The listing builds one solid part. Answer for the finished solid, in the listing's coordinates (mm). A direction names the side the tool comes from. Round coordinates to 2 decimals unless told otherwise and drop trailing zeros. Order: outer loops, then holes, each group sorted by start corner. A loop starts at its lowest first (then second) coordinate and runs counter-clockwise, first axis right, second up. Notation, with made-up numbers: (-34.5, -2.5) -> (-22.5, -2.5) arc R13 ccw to (-22.5, 17.5) -> close; hole circle Ø3 at (75.5, 30.25). An arc over 180 degrees is marked (long way). Answer in a Markdown table with one row per item. Add a question column.
```python
from build123d import *

# Parameters (mm, degrees)
SKETCH1_W           = 36
SKETCH1_H           = 29
BOSS_EXTRUDE1_DEPTH = 1.5
FILLET1_R           = 0.8
SKETCH2_W           = 20
SKETCH2_H           = 1
BOSS_EXTRUDE2_DEPTH = 3


with BuildPart() as part:
    # Sketch1 → Boss-Extrude1 (new body)
    with BuildSketch(Plane(origin=(0, 0, 0), x_dir=(1, 0, 0), z_dir=(0, 1, 0))):
        with Locations((18, -14.5)):
            Rectangle(SKETCH1_W, SKETCH1_H)
    extrude(amount=BOSS_EXTRUDE1_DEPTH)

    # Fillet1
    fillet1_edges = [part.edges().sort_by_distance(p)[0] for p in [
        (0, 0.75, 0),
        (36, 0.75, 0),
        (36, 0.75, 29),
        (0, 0.75, 29),
    ]]
    fillet(fillet1_edges, radius=FILLET1_R)

    # Sketch2 → Boss-Extrude2 (add)
    with BuildSketch(Plane(origin=(0, 1.5, 0), x_dir=(1, 0, 0), z_dir=(0, 1, 0))):
        with Locations((18, -2)):
            Rectangle(SKETCH2_W, SKETCH2_H)
        with Locations((18, -27)):
            Rectangle(SKETCH2_W, SKETCH2_H)
    extrude(amount=BOSS_EXTRUDE2_DEPTH)


solid = part.part
```
Item 1: Find the intervals of material crossed by probe 1 along Z at (x, y) = (26, 2.6); probe 2 along X at (y, z) = (2.3, 27.25); probe 3 along Y at (x, z) = (18, 4), in increasing order. Write a range as [from, to].
Item 2: The part is cut by section A-A, the plane y = 2.75. Give the vertices of the cut face in (x, z).
Item 3: A tool of negligible diameter and unlimited length cuts with its end or side. For faces 1 (the face through (28, 3, 27)), 2 (the face through (18, 0, 14)), 3 (the face through (35.77, 0.76, 0.24)), 4 (the face through (18, 3, 2.5)), 5 (the face through (8, 3, 2)), from which of +Z, -Z, +X, -X, +Y, -Y can it reach the whole face along a straight path? Write none if from no direction.
Item 4: For a pull along Z with two mould halves and no side action, classify faces 6 (the face through (18, 1.5, 14)), 7 (the face through (18, 3, 27.5)), 8 (the face through (0, 1, 15)) as released by +Z, released by -Z, zero draft, split by the parting line, or undercut.
Item 5: The part is cut by section C-C, the plane z = 7. Give the vertices of the cut face in (x, y), and give its area (3 significant figures).
Item 6: The part is cut by section D-D, the plane x = 30. Give the vertices of the cut face in (y, z).
Item 7: Flat-ended cylindrical pins translate along their axes: P1, Ø0.8, axis at y = 3.5, z = 27, coming from the +X side; P2, Ø2.5, axis at x = 20, y = 2.5, coming from the -Z side; P3, Ø6, axis at x = 15, z = 13, coming from the +Y side; P4, Ø0.9, axis at x = 15.5, y = 2.5, coming from the +Z side. Find the tip coordinate at first contact, or state that the pin passes through.
Item 8: The part is cut by section B-B, the plane x = 14. Give the vertices of the cut face in (y, z).
Resolved:
| question | item | result |
|---|---|---|
| 1 | probe 1 | [1.5, 2.5], [26.5, 27.5] |
| 1 | probe 2 | [8, 28] |
| 1 | probe 3 | [0, 1.5] |
| 2 | outline | (8, 1.5) -> (28, 1.5) -> (28, 2.5) -> (8, 2.5) -> close; (8, 26.5) -> (28, 26.5) -> (28, 27.5) -> (8, 27.5) -> close |
| 3 | face 1 | +Z, -Z, +X, +Y |
| 3 | face 2 | +Z, -Z, +X, -X, -Y |
| 3 | face 3 | -Z, +X, +Y, -Y |
| 3 | face 4 | +X, -X, +Y |
| 3 | face 5 | +Z, -Z, -X, +Y |
| 4 | face 6 | undercut |
| 4 | face 7 | released by +Z |
| 4 | face 8 | zero draft |
| 5 | outline | (0, 0) -> (36, 0) -> (36, 1.5) -> (0, 1.5) -> close |
| 5 | area | 54.0 mm2 |
| 6 | outline | (0, 0) -> (1.5, 0) -> (1.5, 29) -> (0, 29) -> close |
| 7 | P1 | x = 28 |
| 7 | P2 | z = 0 |
| 7 | P3 | y = 1.5 |
| 7 | P4 | z = 27.5 |
| 8 | outline | (0, 0) -> (1.5, 0) -> (1.5, 1.5) -> (4.5, 1.5) -> (4.5, 2.5) -> (1.5, 2.5) -> (1.5, 26.5) -> (4.5, 26.5) -> (4.5, 27.5) -> (1.5, 27.5) -> (1.5, 29) -> (0, 29) -> close |
